The model under review builds one solid part; all positions refer to its coordinate system, in mm. Round coordinates to 2 decimals unless told otherwise and drop trailing zeros. Loops run counter-clockwise (first coordinate to the right, second up) from the corner with the lowest first, then second, coordinate; pieces in that order, holes last. Notation, with made-up numbers: (41, -18.5) -> (63, -18.5) arc R13 ccw to (63, -4.5) -> close; hole circle Ø1 at (-26.5, 46). An arc over 180 degrees is marked (long way). Write each question's results on one line, items separated by ' | '. Start each with the question number.
Item 1: We need section A-A (y = -4). Give the boundary of the cut face in (x, z), and give its area (4 significant figures).
Item 2: We need section D-D (z = 37.5). Give the boundary of the cut face in (x, y).
Item 3: We need section B-B (y = -16.5). Give the boundary of the cut face in (x, z).
Item 4: We need section C-C (x = 0.7). Give the number of separate pieces and of enclosed holes in the cut face, and give its area (3 significant figures).
Item 5: Clearance check with flat-ended pins moving along their axes: pin 1 Ø8 at (y, z) = (-12.5, 0) entering from +X; pin 2 Ø0.9 at (x, y) = (2, 16) entering from +Z; pin 3 Ø1.5 at (x, z) = (1.5, 48) entering from +Y; pin 4 Ø0.9 at (x, z) = (1.5, 38.5) entering from -Y. State where each tip first meets the part, or that it passes through.
Item 6: For L1, parallel to Z at x = 1.15, y = -21; L2, parallel to Y at x = 0.6, z = -0.5; L3, parallel to Y at x = 0.2, z = 8, list the stretches that pass through material, from the lowest coordinate up. Write a range as from..to.
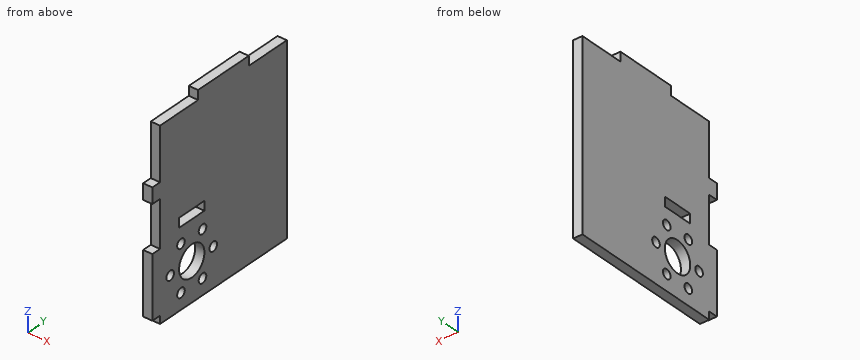
Autodesk Inventor part; units mm, degrees
ref_plane "YZ Plane" through (0, 0, 0) normal (1, 0, 0) x (0, 1, 0)
ref_plane "XZ Plane" through (0, 0, 0) normal (0, 1, 0) x (-1, 0, 0)
ref_plane "XY Plane" through (0, 0, 0) normal (0, 0, 1) x (1, 0, 0)
sketch "Sketch1" plane through (0, 0, 0) normal (1, 0, 0) x (0, 1, 0)
  line L0 (25, -12.5) -> (-25, -12.5)
  line L1 (-25, -12.5) -> (-25, 50)
  line L2 (-25, 50) -> (25, 50)
  line L3 (25, 50) -> (25, -12.5)
  circle A0 centre (-12.5, 0) radius 12.5 construction
  circle A1 centre (-12.5, 0) radius 5
  point P0 (0, 0)
  point P1 (0, -12.5)
  dimension "d0" = 50
  dimension "d1" = 50
  dimension "d2" = 25
  dimension "d3" = 12.5
  dimension "d4" = 10
extrude "Extrusion1" add sketch "Sketch1" along normal blind 3
sketch "Sketch2" plane through (0, 0, 0) normal (-1, 0, 0) x (0, 0, 1)
  line L0 (-10, -25) -> (10, -25)
  line L1 (10, -25) -> (10, -28)
  line L2 (10, -28) -> (-10, -28)
  line L3 (-10, -28) -> (-10, -25)
  line L4 (50, -25) -> (-12.5, -25)
  line L5 (25, -25) -> (30, -25)
  line L6 (30, -25) -> (30, -28)
  line L7 (30, -28) -> (25, -28)
  line L8 (25, -28) -> (25, -25)
  point P0 (0, 0)
  point P1 (0, -28)
  dimension "d7" = 20
  dimension "d8" = 3
  dimension "d9" = 5
  dimension "d10" = 3
  dimension "d11" = 15
extrude "Extrusion2" add sketch "Sketch2" against normal blind 3
sketch "Sketch3" plane through (0, 0, 0) normal (-1, 0, 0) x (0, 0, 1)
  line L0 (50, -25) -> (47, -25)
  line L1 (47, -25) -> (47, -10)
  line L2 (47, -10) -> (50, -10)
  line L3 (50, -10) -> (50, -25)
  line L4 (50, 25) -> (47, 25)
  line L5 (47, 25) -> (47, 10)
  line L6 (47, 10) -> (50, 10)
  line L7 (50, 10) -> (50, 25)
  point P0 (0, 0)
  dimension "d14" = 20
  dimension "d15" = 10
  dimension "d16" = 3
extrude "Extrusion3" cut sketch "Sketch3" against normal blind 3
sketch "Sketch4" plane through (0, 0, 0) normal (-1, 0, 0) x (0, 0, 1)
  circle A0 centre (0, -12.5) radius 5
  circle A1 centre (0, -4) radius 1.5
  point P0 (0, 0)
  dimension "d19" = 3
  dimension "d20" = 8.5
extrude "Extrusion4" cut sketch "Sketch4" against normal blind 3 contours A1
pattern_circular "Circular Pattern1" count 6 over 360 about axis through (0, -12.5, 0) along (1, 0, 0) of "Extrusion4"
sketch "Sketch5" plane through (0, 0, 0) normal (-1, 0, 0) x (0, 0, 1)
  circle A0 centre (0, -12.5) radius 5
  circle A1 centre (0, -12.5) radius 12.5 construction
  line L0 (12.5, -7.5) -> (15.5, -7.5)
  line L1 (15.5, -7.5) -> (15.5, -17.5)
  line L2 (15.5, -17.5) -> (12.5, -17.5)
  line L3 (12.5, -17.5) -> (12.5, -7.5)
  point P0 (0, 0)
  point P1 (12.5, -12.5)
  dimension "d26" = 25
  dimension "d27" = 3
  dimension "d28" = 10
extrude "Extrusion5" cut sketch "Sketch5" against normal blind 3 contours L0 L1 L2 L3
properties part number "Motor support"
Here are the results:
1) outline: (0, -12.5) -> (3, -12.5) -> (3, -1.5) -> (0, -1.5) -> close; (0, 1.5) -> (3, 1.5) -> (3, 50) -> (0, 50) -> close | area: 178.5 mm2
2) outline: (0, -25) -> (3, -25) -> (3, 25) -> (0, 25) -> close
3) outline: (0, -12.5) -> (3, -12.5) -> (3, -8.84) -> (0, -8.84) -> close; (0, -5.88) -> (3, -5.88) -> (3, -3) -> (0, -3) -> close; (0, 3) -> (3, 3) -> (3, 5.88) -> (0, 5.88) -> close; (0, 8.84) -> (3, 8.84) -> (3, 12.5) -> (0, 12.5) -> close; (0, 15.5) -> (3, 15.5) -> (3, 47) -> (0, 47) -> close
4) separate pieces: 1 | enclosed holes: 8 | area: 2,960 mm2
5) pin 1: passes through | pin 2: stops at z = 47 | pin 3: stops at y = 10 | pin 4: stops at y = -25
6) L1: z = -12.5..-1.5, 1.5..47 | L2: y = -28..-22.41, -19.59..-17.47, -7.53..-5.41, -2.59..25 | L3: y = -28..-18.11, -15.39..-9.61, -6.89..25
